```python
from build123d import *

# Parameters (mm, degrees)
F0_R     = 10.925
F0_R_2   = 1.5
F0_R_3   = 5
F1_DEPTH = 3.8
F0_R_4   = 3.5
F2_DEPTH = 5.3
F3_DEPTH = 9.9
F4_SIZE  = 1
F5_SIZE  = 0.2


with BuildPart() as f1:
    # F0 (on Top) → F1 (new body)
    with BuildSketch(Plane.XY):
        Circle(F0_R)
        with Locations((-5.656854, -5.656854)):
            Circle(F0_R_2, mode=Mode.SUBTRACT)
        with Locations((5.656854, -5.656854)):
            Circle(F0_R_2, mode=Mode.SUBTRACT)
        with Locations((-5.656854, 5.656854)):
            Circle(F0_R_2, mode=Mode.SUBTRACT)
        Circle(F0_R_3, mode=Mode.SUBTRACT)
        with Locations((5.656854, 5.656854)):
            Circle(F0_R_2, mode=Mode.SUBTRACT)
    extrude(amount=F1_DEPTH)

    # F0 (on Top) → F2 (join)
    with BuildSketch(Plane.XY):
        Circle(F0_R_3)
        Circle(F0_R_4, mode=Mode.SUBTRACT)
    extrude(amount=F2_DEPTH)

    # F0 (on Top) → F3 (join)
    with BuildSketch(Plane.XY):
        Circle(F0_R_3)
        Circle(F0_R_4, mode=Mode.SUBTRACT)
    extrude(amount=-F3_DEPTH)

    # F4
    f4_edges = [f1.edges().sort_by_distance(p)[0] for p in [
        (-3.5, 0, 5.3),
        (-3.5, 0, -9.9),
    ]]
    chamfer(f4_edges, length=F4_SIZE)

    # F5
    f5_edges = [f1.edges().sort_by_distance(p)[0] for p in [
        (-7.156854, 5.656854, 3.8),
        (-7.156854, -5.656854, 3.8),
        (4.156854, -5.656854, 3.8),
        (4.156854, 5.656854, 3.8),
        (-10.925, 0, 3.8),
        (-10.925, 0, 0),
    ]]
    chamfer(f5_edges, length=F5_SIZE)


solid = f1.part
```
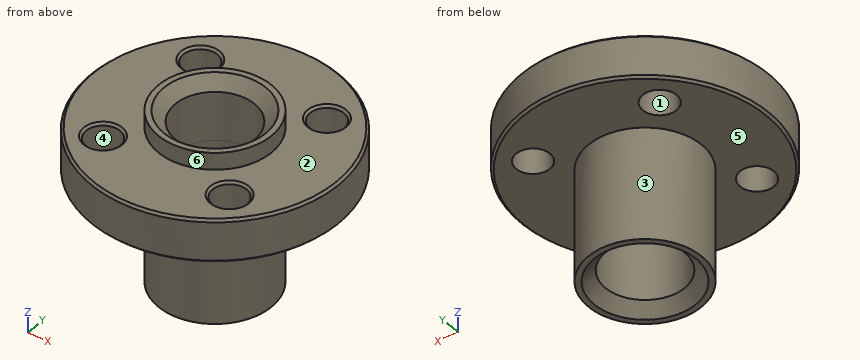
Geometry: final body of the model. Coordinates: model frame, mm. Face numbers are marked on the shaded views. A direction names the side the tool comes from. Round coordinates to 2 decimals unless told otherwise and drop trailing zeros. Write each loop counter-clockwise with the first axis right and the second up, starting at its lowest first coordinate (ties: lowest second). Pieces come first, ordered by that corner, then holes.
Item 1: Section query D-D (z = 2.25). Return loops of the section in (x, y) (3 decimals).
Item 2: Section query A-A (y = 0). Return loops of the section in (x, z) (3 decimals), plus the area to 4 significant figures.
Item 3: Section query C-C (z = -7.75). Return loops of the section in (x, y).
Item 4: Pin query (flat end, axial travel): P1, Ø8, axis at y = 0, z = -0.5, coming from the -X side (3 decimals); P2, Ø6, axis at x = 6, y = -6.5, coming from the -Z side; P3, Ø1.5, axis at y = -3.5, z = 0.5, coming from the -X side; P4, Ø6.5, axis at x = 0.5, y = -0.5, coming from the +Z side. Return the tip coordinate at first contact, or that it passes through.
Item 5: Material intervals for L1, parallel to Y at x = 0, z = -4.5; L2, parallel to Z at x = 1.75, y = -6.25; L3, parallel to Y at x = 5.25, z = 0.25, sorted ascending.
Item 6: Mould query, pull axis Y, two halves, no side actions, for the marked faces 1, 2 and 3. Classes: +Y half, -Y half, draft (parallel to the pull), parting line (faces both ways), or undercut.
Item 7: Set-up query: the marked faces 4, 5 and 6. Return all of +Z, -Z, +X, -X, +Y, -Y with unobstructed straight access to the full face (end or side cutting, diameter ignored); none if empty.
Completed:
1. outline: circle Ø21.85 at (0, 0); hole circle Ø3 at (-5.657, -5.657); hole circle Ø3 at (-5.657, 5.657); hole circle Ø7 at (0, 0); hole circle Ø3 at (5.657, -5.657); hole circle Ø3 at (5.657, 5.657)
2. outline: (-10.925, 0.2) - (-10.725, 0) - (-5, 0) - (-5, -9.9) - (-4.5, -9.9) - (-3.5, -8.9) - (-3.5, 4.3) - (-4.5, 5.3) - (-5, 5.3) - (-5, 3.8) - (-10.725, 3.8) - (-10.925, 3.6) - close; (3.5, -8.9) - (4.5, -9.9) - (5, -9.9) - (5, 0) - (10.725, 0) - (10.925, 0.2) - (10.925, 3.6) - (10.725, 3.8) - (5, 3.8) - (5, 5.3) - (4.5, 5.3) - (3.5, 4.3) - close
2. area: 88.55 mm2
3. outline: circle Ø10 at (0, 0); hole circle Ø7 at (0, 0)
4. P1: stops at x = -10.925
4. P2: stops at z = 0
4. P3: stops at x = -10.57
4. P4: stops at z = 4.76
5. L1: y = -5 to -3.5, 3.5 to 5
5. L2: z = 0 to 3.8
5. L3: y = -9.58 to -7.1, -4.21 to 4.21, 7.1 to 9.58
6. face 1: undercut
6. face 2: draft
6. face 3: parting line
7. face 4: +Z, -Z
7. face 5: -Z
7. face 6: +Z
